```python
from build123d import *

# Parameters (mm, degrees)
SKETCH1_R           = 2.1463
BOSS_EXTRUDE1_DEPTH = 152.4
SKETCH2_W           = 30.13801893
SKETCH2_H           = 25.969901185
CUT_EXTRUDE1_DEPTH  = 152.4


with BuildPart() as part:
    # Sketch1 → Boss-Extrude1 (new body, symmetric)
    with BuildSketch(Plane.XY):
        with BuildLine():
            Line((-9.9949, 7.9883), (-9.9949, 3.2893))
            ThreePointArc((-9.9949, 3.2893), (-9.76427588, 2.73252412), (-9.2075, 2.5019))
            Line((-9.2075, 2.5019), (-8.4963, 2.5019))
            ThreePointArc((-8.4963, 2.5019), (-8.280773853, 2.591173853), (-8.1915, 2.8067))
            Line((-8.1915, 2.8067), (-8.1915, 4.9149))
            ThreePointArc((-8.1915, 4.9149), (-7.674065253, 5.689295824), (-6.760603096, 5.507596904))
            Line((-6.760603096, 5.507596904), (-4.505765747, 3.252759555))
            ThreePointArc((-4.505765747, 3.252759555), (-3.856054457, 2.280397894), (-3.627906192, 1.133419111))
            Line((-3.627906192, 1.133419111), (-3.627906192, -1.133419111))
            ThreePointArc((-3.627906192, -1.133419111), (-3.856054457, -2.280397894), (-4.505765747, -3.252759555))
            Line((-4.505765747, -3.252759555), (-6.760603096, -5.507596904))
            ThreePointArc((-6.760603096, -5.507596904), (-7.674065253, -5.689295824), (-8.1915, -4.9149))
            Line((-8.1915, -4.9149), (-8.1915, -2.8067))
            ThreePointArc((-8.1915, -2.8067), (-8.280773853, -2.591173853), (-8.4963, -2.5019))
            Line((-8.4963, -2.5019), (-9.2075, -2.5019))
            ThreePointArc((-9.2075, -2.5019), (-9.76427588, -2.73252412), (-9.9949, -3.2893))
            Line((-9.9949, -3.2893), (-9.9949, -7.9883))
            ThreePointArc((-9.9949, -7.9883), (-9.407180467, -9.407180467), (-7.9883, -9.9949))
            Line((-7.9883, -9.9949), (-3.2893, -9.9949))
            ThreePointArc((-3.2893, -9.9949), (-2.73252412, -9.76427588), (-2.5019, -9.2075))
            Line((-2.5019, -9.2075), (-2.5019, -8.4963))
            ThreePointArc((-2.5019, -8.4963), (-2.591173853, -8.280773853), (-2.8067, -8.1915))
            Line((-2.8067, -8.1915), (-4.9149, -8.1915))
            ThreePointArc((-4.9149, -8.1915), (-5.689295824, -7.674065253), (-5.507596904, -6.760603096))
            Line((-5.507596904, -6.760603096), (-3.252759555, -4.505765747))
            ThreePointArc((-3.252759555, -4.505765747), (-2.280397894, -3.856054457), (-1.133419111, -3.627906192))
            Line((-1.133419111, -3.627906192), (1.133419111, -3.627906192))
            ThreePointArc((1.133419111, -3.627906192), (2.280397894, -3.856054457), (3.252759555, -4.505765747))
            Line((3.252759555, -4.505765747), (5.507596904, -6.760603096))
            ThreePointArc((5.507596904, -6.760603096), (5.689295824, -7.674065253), (4.9149, -8.1915))
            Line((4.9149, -8.1915), (2.8067, -8.1915))
            ThreePointArc((2.8067, -8.1915), (2.591173853, -8.280773853), (2.5019, -8.4963))
            Line((2.5019, -8.4963), (2.5019, -9.2075))
            ThreePointArc((2.5019, -9.2075), (2.73252412, -9.76427588), (3.2893, -9.9949))
            Line((3.2893, -9.9949), (7.9883, -9.9949))
            ThreePointArc((7.9883, -9.9949), (9.407180467, -9.407180467), (9.9949, -7.9883))
            Line((9.9949, -7.9883), (9.9949, -3.2893))
            ThreePointArc((9.9949, -3.2893), (9.76427588, -2.73252412), (9.2075, -2.5019))
            Line((9.2075, -2.5019), (8.4963, -2.5019))
            ThreePointArc((8.4963, -2.5019), (8.280773853, -2.591173853), (8.1915, -2.8067))
            Line((8.1915, -2.8067), (8.1915, -4.9149))
            ThreePointArc((8.1915, -4.9149), (7.674065253, -5.689295824), (6.760603096, -5.507596904))
            Line((6.760603096, -5.507596904), (4.505765747, -3.252759555))
            ThreePointArc((4.505765747, -3.252759555), (3.856054457, -2.280397894), (3.627906192, -1.133419111))
            Line((3.627906192, -1.133419111), (3.627906192, 1.133419111))
            ThreePointArc((3.627906192, 1.133419111), (3.856054457, 2.280397894), (4.505765747, 3.252759555))
            Line((4.505765747, 3.252759555), (6.760603096, 5.507596904))
            ThreePointArc((6.760603096, 5.507596904), (7.674065253, 5.689295824), (8.1915, 4.9149))
            Line((8.1915, 4.9149), (8.1915, 2.8067))
            ThreePointArc((8.1915, 2.8067), (8.280773853, 2.591173853), (8.4963, 2.5019))
            Line((8.4963, 2.5019), (9.2075, 2.5019))
            ThreePointArc((9.2075, 2.5019), (9.76427588, 2.73252412), (9.9949, 3.2893))
            Line((9.9949, 3.2893), (9.9949, 7.9883))
            ThreePointArc((9.9949, 7.9883), (9.407180467, 9.407180467), (7.9883, 9.9949))
            Line((7.9883, 9.9949), (3.2893, 9.9949))
            ThreePointArc((3.2893, 9.9949), (2.73252412, 9.76427588), (2.5019, 9.2075))
            Line((2.5019, 9.2075), (2.5019, 8.4963))
            ThreePointArc((2.5019, 8.4963), (2.591173853, 8.280773853), (2.8067, 8.1915))
            Line((2.8067, 8.1915), (4.9149, 8.1915))
            ThreePointArc((4.9149, 8.1915), (5.689295824, 7.674065253), (5.507596904, 6.760603096))
            Line((5.507596904, 6.760603096), (3.252759555, 4.505765747))
            ThreePointArc((3.252759555, 4.505765747), (2.280397894, 3.856054457), (1.133419111, 3.627906192))
            Line((1.133419111, 3.627906192), (-1.133419111, 3.627906192))
            ThreePointArc((-1.133419111, 3.627906192), (-2.280397894, 3.856054457), (-3.252759555, 4.505765747))
            Line((-3.252759555, 4.505765747), (-5.507596904, 6.760603096))
            ThreePointArc((-5.507596904, 6.760603096), (-5.689295824, 7.674065253), (-4.9149, 8.1915))
            Line((-4.9149, 8.1915), (-2.8067, 8.1915))
            ThreePointArc((-2.8067, 8.1915), (-2.591173853, 8.280773853), (-2.5019, 8.4963))
            Line((-2.5019, 8.4963), (-2.5019, 9.2075))
            ThreePointArc((-2.5019, 9.2075), (-2.73252412, 9.76427588), (-3.2893, 9.9949))
            Line((-3.2893, 9.9949), (-7.9883, 9.9949))
            ThreePointArc((-7.9883, 9.9949), (-9.407180467, 9.407180467), (-9.9949, 7.9883))
        make_face()
        Circle(SKETCH1_R, mode=Mode.SUBTRACT)
    extrude(amount=BOSS_EXTRUDE1_DEPTH, both=True)

    # Sketch2 → Cut-Extrude1 (cut)
    with BuildSketch(Plane.XY.offset(152.4)):
        with Locations((0.230542333, -0.84546573)):
            Rectangle(SKETCH2_W, SKETCH2_H)
    extrude(amount=-CUT_EXTRUDE1_DEPTH, mode=Mode.SUBTRACT)


solid = part.part
```
Source: CAD feature listing. Evaluate the final solid. Frame: model axes, mm. Give positions to 0.01 mm unless a question says otherwise; leave off trailing zeros.
(1) Pull-direction query (X, two-part tool) for faces 1 (the face through (-6, 9.995, -75)), 2 (the face through (-9.995, 6, -75)), 3 (the face through (2.05, 0.64, -77.27)), 4 (the face through (9.995, -6, -75)); classes: +X half, -X half, draft (parallel to the pull), parting line (faces both ways), or undercut.
(2) Contact query for flat-ended pins moving along their axis: P1, Ø1.8, axis at y = 0, z = -101, coming from the -X side; P2, Ø0.6, axis at y = -8.5, z = -57, coming from the -X side; P3, Ø3.5, axis at x = 0, y = 0, coming from the -Z side; P4, Ø0.8, axis at x = 9, z = -66.5, coming from the -Y side. Output: stop coordinate, or through.
(3) Material intervals for line 1 along Y through (x, z) = (0, -121); line 2 along Y through (x, z) = (2.75, -91); line 3 along X through (y, z) = (-5, -64), sorted ascending.
Outcome:
1. face 1: draft
1. face 2: -X half
1. face 3: undercut
1. face 4: +X half
2. P1: stops at x = -3.63
2. P2: stops at x = -9.98
2. P3: passes through
2. P4: stops at y = -9.9
3. line 1: y = -3.63 to -2.15, 2.15 to 3.63
3. line 2: y = -9.78 to -8.2, -4.1 to 4.1, 8.2 to 9.78
3. line 3: x = -9.99 to -8.19, -6.25 to -3.75, 3.75 to 6.25, 8.19 to 9.99
